from build123d import *

# Parameters (mm, degrees)
F1_DEPTH = 6.35


with BuildPart() as f1:
    # F0 (on Top) → F1 (new body)
    with BuildSketch(Plane.XY):
        with BuildLine():
            Line((-54.6100006601, 184.3987628429), (-86.3600006601, 184.3987628429))
            Line((-86.3600006601, 184.3987628429), (-86.3600006601, 139.9487628429))
            Line((-86.3600006601, 139.9487628429), (-81.5975006601, 139.9487628429))
            ThreePointArc((-81.5975006601, 139.9487628429), (-80.0100006601, 141.5362628429), (-78.4225006601, 139.9487628429))
            ThreePointArc((-78.4225006601, 139.9487628429), (-78.887468645, 138.8262308277), (-80.0100006601, 138.3612628429))
            Line((-80.0100006601, 138.3612628429), (-80.0100006601, 122.4862628429))
            ThreePointArc((-80.0100006601, 122.4862628429), (-78.887468645, 122.021294858), (-78.4225006601, 120.8987628429))
            ThreePointArc((-78.4225006601, 120.8987628429), (-80.0100006601, 119.3112628429), (-81.5975006601, 120.8987628429))
            Line((-81.5975006601, 120.8987628429), (-86.3600006601, 120.8987628429))
            Line((-86.3600006601, 120.8987628429), (-86.3600006601, 38.3487628429))
            Line((-86.3600006601, 38.3487628429), (-81.5975006601, 38.3487628429))
            ThreePointArc((-81.5975006601, 38.3487628429), (-80.0100006601, 39.9362628429), (-78.4225006601, 38.3487628429))
            ThreePointArc((-78.4225006601, 38.3487628429), (-78.887468645, 37.2262308277), (-80.0100006601, 36.7612628429))
            Line((-80.0100006601, 36.7612628429), (-80.0100006601, 20.8862628429))
            ThreePointArc((-80.0100006601, 20.8862628429), (-78.887468645, 20.421294858), (-78.4225006601, 19.2987628429))
            ThreePointArc((-78.4225006601, 19.2987628429), (-80.0100006601, 17.7112628429), (-81.5975006601, 19.2987628429))
            Line((-81.5975006601, 19.2987628429), (-86.3600006601, 19.2987628429))
            Line((-86.3600006601, 19.2987628429), (-86.3600006601, -63.2512371571))
            Line((-86.3600006601, -63.2512371571), (-81.5975006601, -63.2512371571))
            ThreePointArc((-81.5975006601, -63.2512371571), (-80.0100006601, -61.6637371571), (-78.4225006601, -63.2512371571))
            ThreePointArc((-78.4225006601, -63.2512371571), (-78.887468645, -64.3737691723), (-80.0100006601, -64.8387371571))
            Line((-80.0100006601, -64.8387371571), (-80.0100006601, -80.7137371571))
            ThreePointArc((-80.0100006601, -80.7137371571), (-78.887468645, -81.178705142), (-78.4225006601, -82.3012371571))
            ThreePointArc((-78.4225006601, -82.3012371571), (-80.0100006601, -83.8887371571), (-81.5975006601, -82.3012371571))
            Line((-81.5975006601, -82.3012371571), (-86.3600006601, -82.3012371571))
            Line((-86.3600006601, -82.3012371571), (-86.3600006601, -126.7512371571))
            Line((-86.3600006601, -126.7512371571), (-54.6100006601, -126.7512371571))
            Line((-54.6100006601, -126.7512371571), (-54.6100006601, -121.9887371571))
            ThreePointArc((-54.6100006601, -121.9887371571), (-55.7325326753, -119.278705142), (-53.0225006601, -120.4012371571))
            Line((-53.0225006601, -120.4012371571), (-37.1475006601, -120.4012371571))
            ThreePointArc((-37.1475006601, -120.4012371571), (-35.5600006601, -118.8137371571), (-33.9725006601, -120.4012371571))
            ThreePointArc((-33.9725006601, -120.4012371571), (-34.437468645, -121.5237691723), (-35.5600006601, -121.9887371571))
            Line((-35.5600006601, -121.9887371571), (-35.5600006601, -126.7512371571))
            Line((-35.5600006601, -126.7512371571), (21.5899993399, -126.7512371571))
            Line((21.5899993399, -126.7512371571), (21.5899993399, -121.9887371571))
            ThreePointArc((21.5899993399, -121.9887371571), (20.4674673247, -119.278705142), (23.1774993399, -120.4012371571))
            Line((23.1774993399, -120.4012371571), (39.0524993399, -120.4012371571))
            ThreePointArc((39.0524993399, -120.4012371571), (40.6399993399, -118.8137371571), (42.2274993399, -120.4012371571))
            ThreePointArc((42.2274993399, -120.4012371571), (41.762531355, -121.5237691723), (40.6399993399, -121.9887371571))
            Line((40.6399993399, -121.9887371571), (40.6399993399, -126.7512371571))
            Line((40.6399993399, -126.7512371571), (97.7899993399, -126.7512371571))
            Line((97.7899993399, -126.7512371571), (97.7899993399, -121.9887371571))
            ThreePointArc((97.7899993399, -121.9887371571), (96.6674673247, -119.278705142), (99.3774993399, -120.4012371571))
            Line((99.3774993399, -120.4012371571), (115.2524993399, -120.4012371571))
            ThreePointArc((115.2524993399, -120.4012371571), (116.8399993399, -118.8137371571), (118.4274993399, -120.4012371571))
            ThreePointArc((118.4274993399, -120.4012371571), (117.962531355, -121.5237691723), (116.8399993399, -121.9887371571))
            Line((116.8399993399, -121.9887371571), (116.8399993399, -126.7512371571))
            Line((116.8399993399, -126.7512371571), (148.5899993399, -126.7512371571))
            Line((148.5899993399, -126.7512371571), (148.5899993399, -82.3012371571))
            Line((148.5899993399, -82.3012371571), (143.8274993399, -82.3012371571))
            ThreePointArc((143.8274993399, -82.3012371571), (141.1174673247, -83.4237691723), (142.2399993399, -80.7137371571))
            Line((142.2399993399, -80.7137371571), (142.2399993399, -64.8387371571))
            ThreePointArc((142.2399993399, -64.8387371571), (141.1174673247, -62.128705142), (143.8274993399, -63.2512371571))
            Line((143.8274993399, -63.2512371571), (148.5899993399, -63.2512371571))
            Line((148.5899993399, -63.2512371571), (148.5899993399, 19.2987628429))
            Line((148.5899993399, 19.2987628429), (143.8274993399, 19.2987628429))
            ThreePointArc((143.8274993399, 19.2987628429), (141.1174673247, 18.1762308277), (142.2399993399, 20.8862628429))
            Line((142.2399993399, 20.8862628429), (142.2399993399, 36.7612628429))
            ThreePointArc((142.2399993399, 36.7612628429), (141.1174673247, 39.471294858), (143.8274993399, 38.3487628429))
            Line((143.8274993399, 38.3487628429), (148.5899993399, 38.3487628429))
            Line((148.5899993399, 38.3487628429), (148.5899993399, 120.8987628429))
            Line((148.5899993399, 120.8987628429), (143.8274993399, 120.8987628429))
            ThreePointArc((143.8274993399, 120.8987628429), (141.1174673247, 119.7762308277), (142.2399993399, 122.4862628429))
            Line((142.2399993399, 122.4862628429), (142.2399993399, 138.3612628429))
            ThreePointArc((142.2399993399, 138.3612628429), (141.1174673247, 141.071294858), (143.8274993399, 139.9487628429))
            Line((143.8274993399, 139.9487628429), (148.5899993399, 139.9487628429))
            Line((148.5899993399, 139.9487628429), (148.5899993399, 184.3987628429))
            Line((148.5899993399, 184.3987628429), (116.8399993399, 184.3987628429))
            Line((116.8399993399, 184.3987628429), (116.8399993399, 179.6362628429))
            ThreePointArc((116.8399993399, 179.6362628429), (117.962531355, 179.171294858), (118.4274993399, 178.0487628429))
            ThreePointArc((118.4274993399, 178.0487628429), (116.8399993399, 176.4612628429), (115.2524993399, 178.0487628429))
            Line((115.2524993399, 178.0487628429), (99.3774993399, 178.0487628429))
            ThreePointArc((99.3774993399, 178.0487628429), (96.6674673247, 176.9262308277), (97.7899993399, 179.6362628429))
            Line((97.7899993399, 179.6362628429), (97.7899993399, 184.3987628429))
            Line((97.7899993399, 184.3987628429), (40.6399993399, 184.3987628429))
            Line((40.6399993399, 184.3987628429), (40.6399993399, 179.6362628429))
            ThreePointArc((40.6399993399, 179.6362628429), (41.762531355, 179.171294858), (42.2274993399, 178.0487628429))
            ThreePointArc((42.2274993399, 178.0487628429), (40.6399993399, 176.4612628429), (39.0524993399, 178.0487628429))
            Line((39.0524993399, 178.0487628429), (23.1774993399, 178.0487628429))
            ThreePointArc((23.1774993399, 178.0487628429), (20.4674673247, 176.9262308277), (21.5899993399, 179.6362628429))
            Line((21.5899993399, 179.6362628429), (21.5899993399, 184.3987628429))
            Line((21.5899993399, 184.3987628429), (-35.5600006601, 184.3987628429))
            Line((-35.5600006601, 184.3987628429), (-35.5600006601, 179.6362628429))
            ThreePointArc((-35.5600006601, 179.6362628429), (-34.437468645, 179.171294858), (-33.9725006601, 178.0487628429))
            ThreePointArc((-33.9725006601, 178.0487628429), (-35.5600006601, 176.4612628429), (-37.1475006601, 178.0487628429))
            Line((-37.1475006601, 178.0487628429), (-53.0225006601, 178.0487628429))
            ThreePointArc((-53.0225006601, 178.0487628429), (-55.7325326753, 176.9262308277), (-54.6100006601, 179.6362628429))
            Line((-54.6100006601, 179.6362628429), (-54.6100006601, 184.3987628429))
        make_face()
    extrude(amount=F1_DEPTH)


solid = f1.part
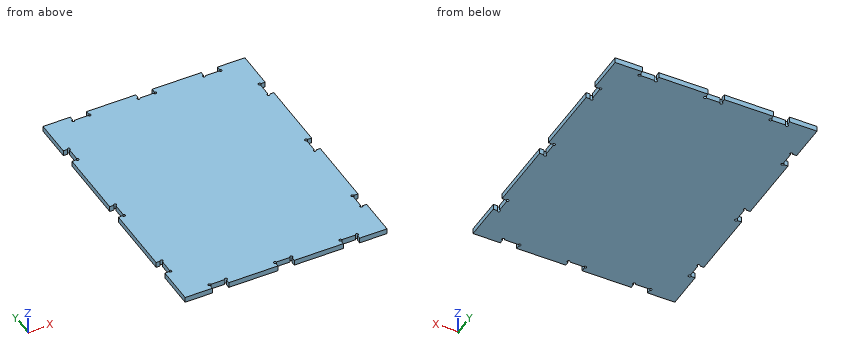
Work out the finished part from the listing and answer in its coordinate system (mm). Round coordinates to 2 decimals unless told otherwise and drop trailing zeros. Loops run counter-clockwise (first coordinate to the right, second up) from the corner with the lowest first, then second, coordinate; pieces in that order, holes last. Notation, with made-up numbers: M -40,33.25 L -35,33.25 A11 ccw -35,37.25 Z; hole C 21.5,-24.5 d4. An arc over 180 degrees is marked long. One line per question, with ' | ' between items. Start each with the question number.
(1) A cutting plane is placed at A-A on x = -48.5. Write down the section's boundary in (y, z).
(2) Flat-ended cylindrical pins translate along their axes: pin 1 Ø1 at (x, y) = (48, 18.5) entering from -Z; pin 2 Ø3 at (y, z) = (130.5, 3) entering from +X; pin 3 Ø1.9 at (x, z) = (110, 2.5) entering from -Y. Find the tip coordinate at first contact, or state that the pin passes through.
(3) Find the intervals of material crossed by line 1 (Y direction, x = 39.5, z = 5.5), in increasing order.
Geometry check:
1) outline: M -120.4,0 L 178.05,0 L 178.05,6.35 L -120.4,6.35 Z
2) pin 1: stops at z = 0 | pin 2: stops at x = 142.24 | pin 3: stops at y = -120.4
3) line 1: y = -119.3 to 176.94
